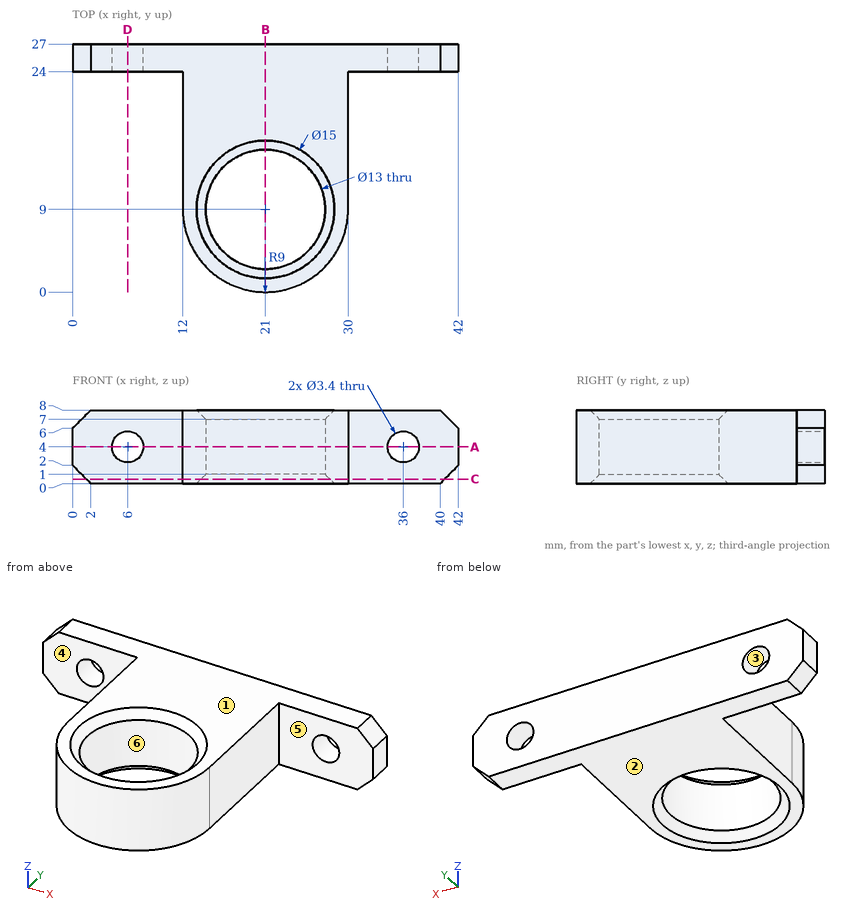
Study the drawing (mm; zero at the part's minimum x, y, z) and answer. A direction names the side the tool comes from. Give positions to 0.01 mm unless a question says otherwise; leave off trailing zeros. Loops run counter-clockwise (first coordinate to the right, second up) from the corner with the lowest first, then second, coordinate; pieces in that order, holes last. Notation, with made-up numbers: (11, 12.25) - (53, 12.25) arc R20 cw to (53, 26.25) - close; hole circle Ø8 at (26.25, 58). An arc over 180 degrees is marked (long way). Use CSV: the item, a comma, the result in double quotes. Start each with the question number.
(1) Find section D-D, the plane x = 6. Determine the outline of the cut face in (y, z), plus the area to 3 significant figures.
(2) Find section A-A, the plane z = 4. Determine the outline of the cut face in (x, y).
(3) Find section C-C, the plane z = 0.5. Determine the outline of the cut face in (x, y), plus the area to 3 significant figures.
(4) Find section B-B, the plane x = 21. Determine the outline of the cut face in (y, z), plus the area to 3 significant figures.
(5) A tool of negligible diameter and unlimited length cuts with its end or side. For the marked faces 4, 5 and 6, from which of +Z, -Z, +X, -X, +Y, -Y can it reach the whole face along a straight path? Write none if from no direction.
(6) Find the intervals of material crossed by L1, parallel to X at y = 25.3, z = 4; L2, parallel to Z at x = 6, y = 26.3; L3, parallel to Y at x = 21, z = 2.8, in increasing order.
(7) Each of these flat-tipped pins is pushed along its axis until it touches: pin 1 (1 mm diameter, centred on y = 14, z = 3, fed in from -X); pin 2 (2.5 mm diameter, centred on y = 14, z = 3, fed in from +X); pin 3 (1 mm diameter, centred on x = 24.5, z = 3, fed in from -Y). Where does it stop, or does it pass through?
(8) Determine the mould class of the marked faces 1, 2 and 3 for opening direction Z: released by +Z, released by -Z, zero draft, split by the parting line, or undercut.
Results found:
1,outline,"(24, 0) - (27, 0) - (27, 2.3) - (24, 2.3) - close; (24, 5.7) - (27, 5.7) - (27, 8) - (24, 8) - close"
1,area,"13.8 mm^2"
2,outline,"(0, 24) - (4.3, 24) - (4.3, 27) - (0, 27) - close; (7.7, 24) - (12, 24) - (12, 9) arc R9 ccw to (30, 9) - (30, 24) - (34.3, 24) - (34.3, 27) - (7.7, 27) - close; (37.7, 24) - (42, 24) - (42, 27) - (37.7, 27) - close; hole circle Ø13 at (21, 9)"
3,outline,"(1.5, 24) - (12, 24) - (12, 9) arc R9 ccw to (30, 9) - (30, 24) - (40.5, 24) - (40.5, 27) - (1.5, 27) - close; hole circle Ø14 at (21, 9)"
3,area,"360 mm^2"
4,outline,"(0, 0) - (1.5, 0) - (2.5, 1) - (2.5, 7) - (1.5, 8) - (0, 8) - close; (15.5, 1) - (16.5, 0) - (27, 0) - (27, 8) - (16.5, 8) - (15.5, 7) - close"
4,area,"110 mm^2"
5,face 4,"+Z, -Z, -X, -Y"
5,face 5,"+Z, -Z, +X, -Y"
5,face 6,"+Z, -Z"
6,L1,"0 to 4.3, 7.7 to 34.3, 37.7 to 42"
6,L2,"0 to 2.3, 5.7 to 8"
6,L3,"0 to 2.5, 15.5 to 27"
7,pin 1,"x = 12"
7,pin 2,"x = 30"
7,pin 3,"y = 0.51"
8,face 1,"released by +Z"
8,face 2,"released by -Z"
8,face 3,"undercut"
